```python
from build123d import *

# Parameters (mm, degrees)
BOSS_EXTRUDE1_DEPTH      = 1.5
BOSS_EXTRUDE1_DEPTH_BACK = 1.5
BOSS_EXTRUDE2_DEPTH      = 1.5
BOSS_EXTRUDE2_DEPTH_BACK = 1.5
SKETCH4_W                = 11.052180397
SKETCH4_H                = 1.65
SKETCH5_R                = 1.4
BOSS_EXTRUDE20_DEPTH     = 3.5
SKETCH6_R                = 26
SKETCH6_R_2              = 25
CUT_EXTRUDE1_DEPTH       = 1.65


with BuildPart() as part:
    # Sketch1 → Revolve1 (revolve)
    with BuildSketch(Plane.XY):
        with BuildLine():
            Line((-20.885, 0), (-20.885, 11.793939121))
            ThreePointArc((-20.885, 11.793939121), (-12.091372858, 20.714220415), (0, 23.985))
            Line((0, 23.985), (0, 25.485))
            ThreePointArc((0, 25.485), (-18.020616319, 18.020616319), (-25.485, 0))
            Line((-25.485, 0), (-24.285, 0))
            Line((-24.285, 0), (-24.285, 0.5))
            Line((-24.285, 0.5), (-22.085, 0.5))
            Line((-22.085, 0.5), (-22.085, 0))
            Line((-22.085, 0), (-20.885, 0))
        make_face()
    revolve(axis=Axis((0, 0, 0), (0, 1, 0)))



with BuildPart() as body_2:
    # Sketch2 → Boss-Extrude1 (new body, two sides)
    with BuildSketch(Plane.XY) as boss_extrude1_sk:
        with BuildLine():
            Line((-24.9, 0), (-35, 0))
            ThreePointArc((-35, 0), (0, 35), (35, 0))
            Line((35, 0), (24.9, 0))
            ThreePointArc((24.9, 0), (0, 24.9), (-24.9, 0))
        make_face()
    extrude(amount=BOSS_EXTRUDE1_DEPTH)
    extrude(boss_extrude1_sk.sketch, amount=-BOSS_EXTRUDE1_DEPTH_BACK)

    # Sketch3 → Boss-Extrude2 (add, two sides)
    with BuildSketch(Plane(origin=(0, 0, 0), x_dir=(0, 0, -1), z_dir=(1, 0, 0))) as boss_extrude2_sk:
        with BuildLine():
            Line((35, 0), (24.9, 0))
            ThreePointArc((24.9, 0), (0, 24.9), (-24.9, 0))
            Line((-24.9, 0), (-35, 0))
            ThreePointArc((-35, 0), (0, 35), (35, 0))
        make_face()
    extrude(amount=BOSS_EXTRUDE2_DEPTH)
    extrude(boss_extrude2_sk.sketch, amount=-BOSS_EXTRUDE2_DEPTH_BACK)

    # Sketch4 → Cut-Revolve2 (revolve, cut)
    with BuildSketch(Plane.XY):
        with Locations((-30.371361379, 0.825)):
            Rectangle(SKETCH4_W, SKETCH4_H)
    revolve(axis=Axis((0, 0, 0), (0, 1, 0)), mode=Mode.SUBTRACT)


with BuildPart() as part_1:
    add(part.part)

    add(body_2.part)  # Boss-Extrude20 merges body 2
    # Sketch5 → Boss-Extrude20 (add)
    with BuildSketch(Plane.XZ.offset(-1.65)):
        with BuildLine():
            Line((-32.23863084, -1.5), (-24.23863084, -1.5))
            ThreePointArc((-24.23863084, -1.5), (-23.660511509, -5.471875377), (-22.4360777, -9.294280094))
            ThreePointArc((-22.4360777, -9.294280094), (-27.026694315, -8.998446643), (-30.695451754, -6.223289498))
            ThreePointArc((-30.695451754, -6.223289498), (-31.843056108, -3.984495189), (-32.23863084, -1.5))
        make_face()
        with Locations((-28.212839525, -4.2)):
            Circle(SKETCH5_R, mode=Mode.SUBTRACT)
        with BuildLine():
            Line((24.23863084, 1.5), (32.23863084, 1.5))
            ThreePointArc((32.23863084, 1.5), (31.843056108, 3.984495189), (30.695451754, 6.223289498))
            ThreePointArc((30.695451754, 6.223289498), (27.026694315, 8.998446643), (22.4360777, 9.294280094))
            ThreePointArc((22.4360777, 9.294280094), (23.660511509, 5.471875377), (24.23863084, 1.5))
        make_face()
        with Locations((28.212839525, 4.2)):
            Circle(SKETCH5_R, mode=Mode.SUBTRACT)
        with BuildLine():
            Line((-1.5, 32.23863084), (-1.5, 24.23863084))
            ThreePointArc((-1.5, 24.23863084), (-5.471875377, 23.660511509), (-9.294280094, 22.4360777))
            ThreePointArc((-9.294280094, 22.4360777), (-8.998446643, 27.026694315), (-6.223289498, 30.695451754))
            ThreePointArc((-6.223289498, 30.695451754), (-3.984495189, 31.843056108), (-1.5, 32.23863084))
        make_face()
        with Locations((-4.2, 28.212839525)):
            Circle(SKETCH5_R, mode=Mode.SUBTRACT)
        with BuildLine():
            Line((1.5, -32.23863084), (1.5, -24.23863084))
            ThreePointArc((1.5, -24.23863084), (5.471875377, -23.660511509), (9.294280094, -22.4360777))
            ThreePointArc((9.294280094, -22.4360777), (8.998446643, -27.026694315), (6.223289498, -30.695451754))
            ThreePointArc((6.223289498, -30.695451754), (3.984495189, -31.843056108), (1.5, -32.23863084))
        make_face()
        with Locations((4.2, -28.212839525)):
            Circle(SKETCH5_R, mode=Mode.SUBTRACT)
    extrude(amount=-BOSS_EXTRUDE20_DEPTH)

    # Sketch6 → Cut-Extrude1 (cut)
    with BuildSketch(Plane.XZ):
        Circle(SKETCH6_R)
        Circle(SKETCH6_R_2, mode=Mode.SUBTRACT)
    extrude(amount=-CUT_EXTRUDE1_DEPTH, mode=Mode.SUBTRACT)


solid = part_1.part
```
The listing builds one solid part. Answer for the finished solid, in the listing's coordinates (mm). A direction names the side the tool comes from. Coordinates: 2 decimals unless noted, no trailing zeros. Write each loop counter-clockwise with the first axis right and the second up, starting at its lowest first coordinate (ties: lowest second). Pieces come first, ordered by that corner, then holes.
Q1. Section B-B, the plane x = 4.2 is taken. Write down the section's boundary in (y, z), then the cut area to 3 significant figures.
Returned:
outline: (0, -24.64) - (1.65, -24.64) - (1.65, -26.81) - (5.15, -26.81) - (5.15, -24.6) arc R25.14 ccw to (25.09, -1.5) - (34.75, -1.5) - (34.75, 1.5) - (25.09, 1.5) arc R25.14 ccw to (1.65, 25.08) - (1.65, 24.64) - (0, 24.64) - (0, 23.92) - (0.5, 23.92) - (0.5, 21.68) - (0, 21.68) - (0, 20.46) - (11.79, 20.46) arc R23.61 cw to (11.79, -20.46) - (0, -20.46) - (0, -21.68) - (0.5, -21.68) - (0.5, -23.92) - (0, -23.92) - close; (1.65, -31.77) - (5.15, -31.77) - (5.15, -29.61) - (1.65, -29.61) - close
area: 206 mm2
Q2. Given P1, Ø16.5, axis at x = 12.5, y = 13, coming from the +Z side; P2, Ø2, axis at x = -15, y = 14.5, coming from the +Z side; P3, Ø12, axis at x = -6.5, z = -1.5, coming from the +Y side; P4, Ø1.5, axis at x = 12, z = -23.5, coming from the +Y side, each flat-ended and moving along its own axis, determine where each tip first touches the part or whether it passes through.
Returned:
P1: stops at z = 23.53
P2: stops at z = 15.97
P3: stops at y = 35
P4: passes through
Q3. Find the intervals of material crossed by line 1 along Z through (x, y) = (0, 0.2) (3 decimals); line 2 along Z through (x, y) = (21, 21.5), in increasing order.
Returned:
line 1: z = -25 to -24.285, -22.085 to -20.885, 20.885 to 22.085, 24.285 to 25
line 2: z = -1.5 to 1.5
Q4. Section A-A, the plane z = 4.2 is taken. Write down the section's boundary in (x, y), then the cut area to 3 significant figures.
Returned:
outline: (-25.08, 1.65) - (-24.64, 1.65) - (-24.64, 0) - (-23.92, 0) - (-23.92, 0.5) - (-21.68, 0.5) - (-21.68, 0) - (-20.46, 0) - (-20.46, 11.79) arc R23.61 cw to (20.46, 11.79) - (20.46, 0) - (21.68, 0) - (21.68, 0.5) - (23.92, 0.5) - (23.92, 0) - (24.64, 0) - (24.64, 1.65) - (26.81, 1.65) - (26.81, 5.15) - (24.6, 5.15) arc R25.14 ccw to (1.5, 25.09) - (1.5, 34.75) - (-1.5, 34.75) - (-1.5, 25.09) arc R25.14 ccw to start; (29.61, 1.65) - (31.77, 1.65) - (31.77, 5.15) - (29.61, 5.15) - close
area: 206 mm2
Q5. Section D-D, the plane x = -13 is taken. Write down the section's boundary in (y, z), then the cut area to 3 significant figures.
Returned:
outline: (0, -21.35) - (1.65, -21.35) - (1.65, -21.86) arc R21.92 ccw to (21.87, -1.5) - (32.5, -1.5) - (32.5, 1.5) - (21.87, 1.5) arc R21.92 ccw to (1.65, 21.86) - (1.65, 21.35) - (0, 21.35) - (0, 20.51) - (0.5, 20.51) - (0.5, 17.85) - (0, 17.85) - (0, 16.35) - (11.79, 16.35) arc R20.16 cw to (11.79, -16.35) - (0, -16.35) - (0, -17.85) - (0.5, -17.85) - (0.5, -20.51) - (0, -20.51) - close
area: 205 mm2
Q6. Which of the six approach directions +Z, -Z, +X, -X, +Y, -Y give full straight-line access (tool end or side, diameter ignored) to faces 1 (the flat face through (28, 5.15, 6)), 2 (the flat face through (-10.2, 1.65, -23.1)), 3 (the flat face through (6, 5.15, -28)), 4 (the flat face through (-1.5, 19, -18)), 5 (the flat face through (-5.4, 5.15, 26.7))?
Returned:
face 1: +Z, +X, +Y
face 2: -Y
face 3: -Z, +X, +Y
face 4: -Z, -X, +Y
face 5: +Z, -X, +Y
Q7. Section C-C, the plane y = 30 is taken. Write down the section's boundary in (x, z), then the cut area to 3 significant figures.
Returned:
outline: (-18.03, -1.5) - (-1.5, -1.5) - (-1.5, -18.03) - (1.5, -18.03) - (1.5, -1.5) - (18.03, -1.5) - (18.03, 1.5) - (1.5, 1.5) - (1.5, 18.03) - (-1.5, 18.03) - (-1.5, 1.5) - (-18.03, 1.5) - close
area: 207 mm2
